Geometry: final body of the model. Coordinates: model frame, mm. A direction names the side the tool comes from. Coordinates: 2 decimals unless noted, no trailing zeros. Order: outer loops, then holes, each group sorted by start corner. A loop starts at its lowest first (then second) coordinate and runs counter-clockwise, first axis right, second up. Notation, with made-up numbers: M 66,11.25 L 89,11.25 A35 ccw 89,50.25 Z; hole C 84.25,8 d8. An arc over 180 degrees is marked long. Write item = value, one per line.
from build123d import *

# Parameters (mm, degrees)
PAD_DEPTH    = 41.95
SKETCH001_R  = 2.5
POCKET_DEPTH = 1.6


with BuildPart() as part:
    # Sketch (on XY_Plane of Origin) → Pad (new body, symmetric)
    with BuildSketch(Plane.XY):
        Polygon((0, 2), (0, -2), (-31, -2), (-35, 2), align=None)
    extrude(amount=PAD_DEPTH, both=True)

    # Mirrored: part across YZ


with BuildPart() as part_1:
    add(part.part)
    add(part.part.mirror(Plane.YZ))

    # Sketch001 (on Face2 of Mirrored) → Pocket (cut)
    with BuildSketch(Plane.XZ.offset(2)):
        Circle(SKETCH001_R)
    extrude(amount=-POCKET_DEPTH, mode=Mode.SUBTRACT)


solid = part_1.part
1) Section D-D, the plane z = 12. Return loops of the section in (x, y).
Numbers:
outline = M -35,2 L -31,-2 L 31,-2 L 35,2 Z
2) Line query: L1, parallel to Z at x = 0, y = -1.3; L2, parallel to X at y = -1.1, z = -23; L3, parallel to X at y = -0.25, z = -7. Output: solid intervals per line, ascending.
Numbers:
L1 = -41.95 to -2.5, 2.5 to 41.95
L2 = -31.9 to 31.9
L3 = -32.75 to 32.75
3) Set-up query: faces 4 (the face through (-0.54, -1.21, -2.44)), 5 (the face through (33, 0, 1)). Return all of +Z, -Z, +X, -X, +Y, -Y with unobstructed straight access to the full face (end or side cutting, diameter ignored); none if empty.
Numbers:
face_4 = -Y
face_5 = +Z, -Z, +X, -Y
4) Pin query (flat end, axial travel): pin 1 (2 mm diameter, centred on y = 0.5, z = 9.5, fed in from -X); pin 2 (2 mm diameter, centred on y = -0.5, z = -33, fed in from -X). Return the tip coordinate at first contact, or that it passes through.
Numbers:
pin_1 = -34.5
pin_2 = -33.5
5) Section B-B, the plane z = 0. Return loops of the section in (x, y).
Numbers:
outline = M -35,2 L -31,-2 L -2.5,-2 L -2.5,-0.4 L 2.5,-0.4 L 2.5,-2 L 31,-2 L 35,2 Z
6) Section A-A, the plane x = 0. Return loops of the section in (y, z).
Numbers:
outline = M -2,-41.95 L 2,-41.95 L 2,41.95 L -2,41.95 L -2,2.5 L -0.4,2.5 L -0.4,-2.5 L -2,-2.5 Z
7) Section C-C, the plane y = 0.5. Return loops of the section in (x, z).
Numbers:
outline = M -33.5,-41.95 L 33.5,-41.95 L 33.5,41.95 L -33.5,41.95 Z
8) Mould query, pull axis Z, two halves, no side actions, for faces 1 (the face through (6, -2, 1)), 2 (the face through (0, 0, 41.95)), 3 (the face through (0, -0.4, 0)). Classes: pulls with the +Z half, pulls with the -Z half, needs draft (parallel to the pull), parting line crosses it, or undercut.
Numbers:
face_1 = needs draft
face_2 = pulls with the +Z half
face_3 = undercut
